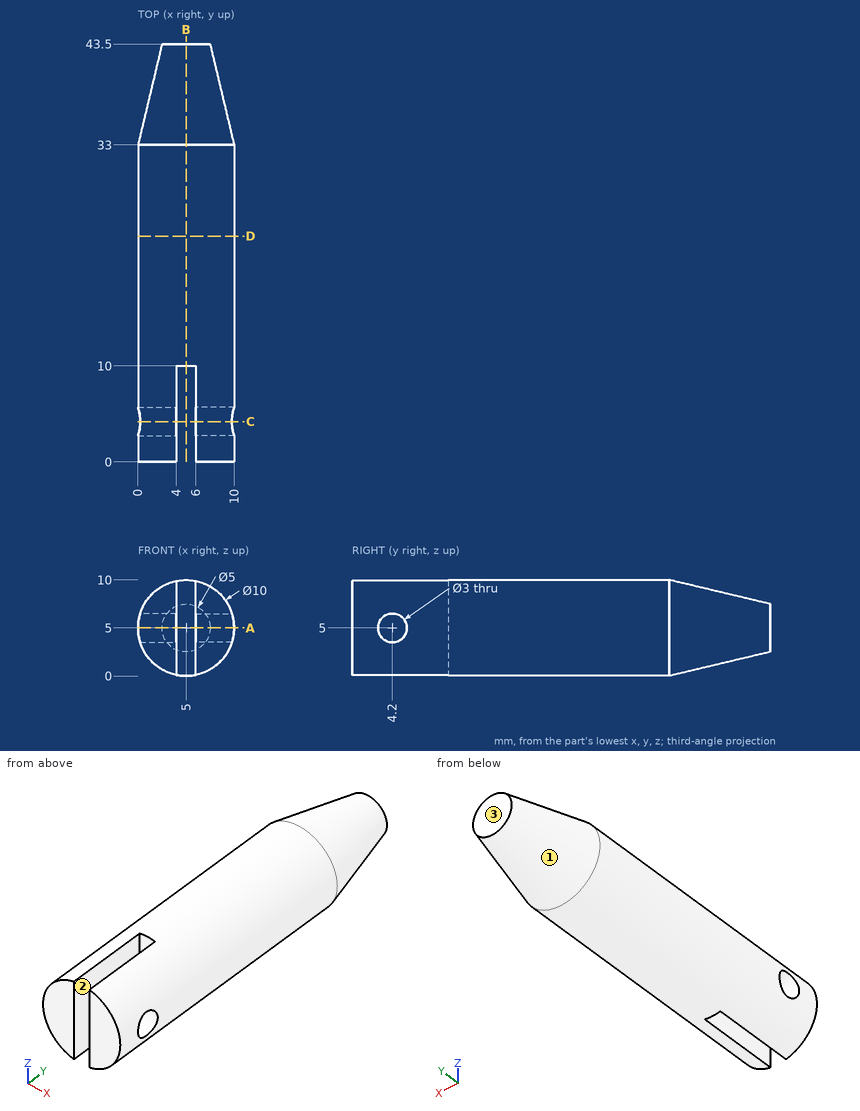
Source: three-view drawing plus pictorial views. Frame: mm from the lowest corner of the part. Round coordinates to 2 decimals unless told otherwise and drop trailing zeros. Loops run counter-clockwise (first coordinate to the right, second up) from the corner with the lowest first, then second, coordinate; pieces in that order, holes last.
Q1. Ray query, line 1 (Y direction, x = 7.4, z = 5); line 2 (Y direction, x = 5.5, z = 7); line 3 (X direction, y = 7, z = 6.25). Return the intervals inside material, ascending.
Q2. First-contact query: P1, Ø2.5, axis at y = 4.2, z = 5, coming from the +X side; P2, Ø0.6, axis at x = 5, z = 7, coming from the -Y side; P3, Ø4, axis at y = 36, z = 5, coming from the +X side; P4, Ø5, axis at x = 1, y = 18.5, coming from the -Z side. Flat tips, straight axial feed; report the tip coordinate or a pass-through.
Q3. Section C-C, the plane y = 4.2. Return loops of the section in (x, z), plus the area to 3 significant figures.
Q4. Section A-A, the plane z = 5. Return loops of the section in (x, y).
Q5. Section D-D, the plane y = 23.5. Return loops of the section in (x, z).
Q6. Section B-B, the plane x = 5. Return loops of the section in (y, z).
Q7. Mould query, pull axis X, two halves, no side actions, for the marked faces 1, 2 and 3. Classes: pulls with the +X half, pulls with the -X half, needs draft (parallel to the pull), parting line crosses it, or undercut.
Solutions:
1. line 1: y = 0 to 2.7, 5.7 to 43.5
1. line 2: y = 10 to 43.5
1. line 3: x = 0.16 to 4, 6 to 9.84
2. P1: passes through
2. P2: stops at y = 10
2. P3: stops at x = 9.76
2. P4: stops at z = 0.23
3. outline: (0.23, 3.5) arc R5 ccw to (4, 0.1) - (4, 3.5) - close; (0.23, 6.5) - (4, 6.5) - (4, 9.9) arc R5 ccw to start; (6, 0.1) arc R5 ccw to (9.77, 3.5) - (6, 3.5) - close; (6, 6.5) - (9.77, 6.5) arc R5 ccw to (6, 9.9) - close
3. area: 35.1 mm2
4. outline: (0, 0) - (4, 0) - (4, 2.7) - (0, 2.7) - close; (0, 5.7) - (4, 5.7) - (4, 10) - (6, 10) - (6, 5.7) - (10, 5.7) - (10, 33) - (7.5, 43.5) - (2.5, 43.5) - (0, 33) - close; (6, 0) - (10, 0) - (10, 2.7) - (6, 2.7) - close
5. outline: circle Ø10 at (5, 5)
6. outline: (10, 0) - (33, 0) - (43.5, 2.5) - (43.5, 7.5) - (33, 10) - (10, 10) - close
7. face 1: parting line crosses it
7. face 2: undercut
7. face 3: needs draft
